Input: part model. Units: mm. Frame: model coordinates. A direction names the side the tool comes from. Round coordinates to 2 decimals unless told otherwise and drop trailing zeros. Write each loop counter-clockwise with the first axis right and the second up, starting at its lowest first coordinate (ties: lowest second). Pieces come first, ordered by that corner, then holes. Notation, with made-up numbers: (32.5, -19.5) - (74.5, -19.5) arc R23 cw to (74.5, 10.5) - close; hole circle Ø7 at (36, 59). An arc over 180 degrees is marked (long way). Use one line per item in the form item = value.
```python
from build123d import *

# Parameters (mm, degrees)
F0_W     = 84.8995
F0_H     = 157.6705
F0_R     = 16.9799
F1_DEPTH = 6.35
F3_DEPTH = 9.525
F5_DEPTH = 9.525


with BuildPart() as f1:
    # F0 (on Top) → F1 (new body)
    with BuildSketch(Plane.XY):
        with Locations((0, -36.3855)):
            Rectangle(F0_W, F0_H)
        Circle(F0_R, mode=Mode.SUBTRACT)
    extrude(amount=-F1_DEPTH)

    # F2 (on face) → F3 (join)
    with BuildSketch(Plane(origin=(-42.44975, 0, 0), x_dir=(0, -1, 0), z_dir=(-1, 0, 0))):
        Polygon((-20.600559, -6.35), (-42.44975, -6.35), (-38.717904, -30.318216), (-29.306301, -28.852831), align=None)
    extrude(amount=-F3_DEPTH)

    # F4 (on face) → F5 (join)
    with BuildSketch(Plane.YZ.offset(42.44975)):
        Polygon((38.717904, -30.318216), (42.44975, -6.35), (20.600559, -6.35), (29.306301, -28.852831), align=None)
    extrude(amount=-F5_DEPTH)


solid = f1.part
```
(1) Material intervals for L1, parallel to Y at x = 0, z = -2; L2, parallel to Z at x = 34, y = -46.5; L3, parallel to X at y = 12, z = -5, sorted ascending.
Derived:
L1 = -115.22 to -16.98, 16.98 to 42.45
L2 = -6.35 to 0
L3 = -42.45 to -12.01, 12.01 to 42.45
(2) Cut plane C-C on x = 27.5. Output: boundary loops of the cut face in (y, z).
Derived:
outline = (-115.22, -6.35) - (42.45, -6.35) - (42.45, 0) - (-115.22, 0) - close
(3) Cut plane B-B on y = 0. Output: boundary loops of the cut face in (x, z), then the cut area to 3 significant figures.
Derived:
outline = (-42.45, -6.35) - (-16.98, -6.35) - (-16.98, 0) - (-42.45, 0) - close; (16.98, -6.35) - (42.45, -6.35) - (42.45, 0) - (16.98, 0) - close
area = 323 mm^2
(4) First-contact query: pin 1 Ø5 at (x, y) = (-31.5, -20) entering from -Z. Flat tip, straight axial feed; report the tip coordinate or a pass-through.
Derived:
pin_1 = -6.35
(5) Cut plane A-A on x = 0. Output: boundary loops of the cut face in (y, z), then the cut area to 3 significant figures.
Derived:
outline = (-115.22, -6.35) - (-16.98, -6.35) - (-16.98, 0) - (-115.22, 0) - close; (16.98, -6.35) - (42.45, -6.35) - (42.45, 0) - (16.98, 0) - close
area = 786 mm^2
(6) Draft query along X for faces 1 (the face through (-42.45, -18, -5)), 2 (the face through (-32.925, 32, -16)), 3 (the face through (37.754, 33.946, -29.575)). Return one class per face: released by +X, released by -X, zero draft, split by the parting line, or undercut.
Derived:
face_1 = released by -X
face_2 = undercut
face_3 = zero draft
(7) Cut plane D-D on y = -88.5. Output: boundary loops of the cut face in (x, z).
Derived:
outline = (-42.45, -6.35) - (42.45, -6.35) - (42.45, 0) - (-42.45, 0) - close
(8) Access query for faces 4 (the face through (-37.75, 40.61, -18.17)), 5 (the face through (32.925, 34, -16)). Directions: +Z, -Z, +X, -X, +Y, -Y. A direction counts if a zero-diameter tool reaches every point of the face in a straight line with its end or side. Return the directions, or none.
Derived:
face_4 = -Z, +X, -X, +Y
face_5 = -Z, +Y, -Y
